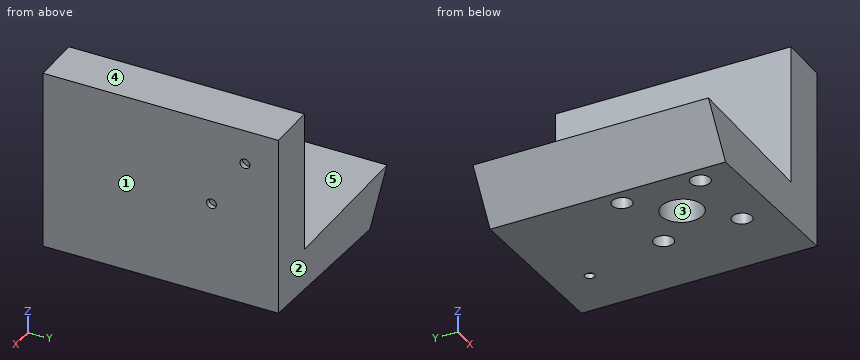
from build123d import *

# Parameters (mm, degrees)
SKETCH1_W           = 41.85
SKETCH1_H           = 10
SKETCH1_W_2         = 10
SKETCH1_H_2         = 29
BOSS_EXTRUDE1_DEPTH = 48
CUT_EXTRUDE1_DEPTH  = 48
SKETCH4_R           = 2
SKETCH4_R_2         = 4.2
CUT_EXTRUDE2_DEPTH  = 48
CUT_EXTRUDE3_DEPTH  = 48
SKETCH6_R           = 1
CUT_EXTRUDE4_DEPTH  = 2
SKETCH7_R           = 1
CUT_EXTRUDE5_DEPTH  = 1
SKETCH8_W           = 65.86504954
SKETCH8_H           = 108.734415267
CUT_EXTRUDE6_DEPTH  = 17.96
BOSS_EXTRUDE2_DEPTH = 17.96
SKETCH10_R          = 1
CUT_EXTRUDE7_DEPTH  = 1
SKETCH11_R          = 1
CUT_EXTRUDE8_DEPTH  = 1


with BuildPart() as part:
    # Sketch1 → Boss-Extrude1 (new body)
    with BuildSketch(Plane(origin=(0, 0, 0), x_dir=(1, 0, 0), z_dir=(0, 1, 0))):
        with Locations((-10.925, 5)):
            Rectangle(SKETCH1_W, SKETCH1_H)
        with Locations((5, -14.5)):
            Rectangle(SKETCH1_W_2, SKETCH1_H_2)
    extrude(amount=BOSS_EXTRUDE1_DEPTH)

    # Sketch3 → Cut-Extrude1 (cut)
    with BuildSketch(Plane(origin=(0, 48, 0), x_dir=(1, 0, 0), z_dir=(0, 1, 0))):
        Polygon((-31.85, 10), (-25.26317425, 10), (-31.85, 0), align=None)
    extrude(amount=-CUT_EXTRUDE1_DEPTH, mode=Mode.SUBTRACT)

    # Sketch4 → Cut-Extrude2 (cut)
    with BuildSketch(Plane.XY):
        with Locations((-5.589559388, 40.980827232)):
            Circle(SKETCH4_R)
        with Locations((-5.629681083, 24.979051073)):
            Circle(SKETCH4_R)
        with Locations((-21.591335547, 41.020948927)):
            Circle(SKETCH4_R)
        with Locations((-21.631457243, 25.019172768)):
            Circle(SKETCH4_R)
        with Locations((-13.629681083, 32.979051073)):
            Circle(SKETCH4_R_2)
    extrude(amount=-CUT_EXTRUDE2_DEPTH, mode=Mode.SUBTRACT)

    # Sketch5 → Cut-Extrude3 (cut)
    with BuildSketch(Plane(origin=(0, 48, 0), x_dir=(1, 0, 0), z_dir=(0, 1, 0))):
        Polygon((-25.26317425, 10), (10, 8), (10, 10), align=None)
    extrude(amount=-CUT_EXTRUDE3_DEPTH, mode=Mode.SUBTRACT)

    # Sketch6 → Cut-Extrude4 (cut)
    with BuildSketch(Plane(origin=(10, 0, 0), x_dir=(0, 0, -1), z_dir=(1, 0, 0))):
        with Locations((-21, 6.391948522)):
            Circle(SKETCH6_R)
        with Locations((-11, 15)):
            Circle(SKETCH6_R)
    extrude(amount=-CUT_EXTRUDE4_DEPTH, mode=Mode.SUBTRACT)

    # Sketch7 → Cut-Extrude5 (cut)
    with BuildSketch(Plane(origin=(0.484340621, 0, -8.539693864), x_dir=(-0.9983954953921488, 0, -0.056625389894163713), z_dir=(0.056625389894163713, 0, -0.9983954953921488))):
        with Locations((10.469048165, 7)):
            Circle(SKETCH7_R)
    extrude(amount=-CUT_EXTRUDE5_DEPTH, mode=Mode.SUBTRACT)

    # Sketch8 → Cut-Extrude6 (cut)
    with BuildSketch(Plane.XZ):
        with Locations((-12.632558392, 5.858470362)):
            Rectangle(SKETCH8_W, SKETCH8_H)
    extrude(amount=-CUT_EXTRUDE6_DEPTH, mode=Mode.SUBTRACT)

    # Sketch9 → Boss-Extrude2 (add)
    with BuildSketch(Plane(origin=(0, 48, 0), x_dir=(1, 0, 0), z_dir=(0, 1, 0))):
        Polygon((10, -29), (0, -29), (0, 0), (-31.85, 0), (-25.26317425, 10), (10, 8), align=None)
    extrude(amount=BOSS_EXTRUDE2_DEPTH)

    # Sketch10 → Cut-Extrude7 (cut)
    with BuildSketch(Plane(origin=(10, 0, 0), x_dir=(0, 0, -1), z_dir=(1, 0, 0))):
        with Locations((-21.942879274, 59.132798009)):
            Circle(SKETCH10_R)
        with Locations((-11.347569505, 52.312182855)):
            Circle(SKETCH10_R)
    extrude(amount=-CUT_EXTRUDE7_DEPTH, mode=Mode.SUBTRACT)

    # Sketch11 → Cut-Extrude8 (cut)
    with BuildSketch(Plane(origin=(0.484340621, 0, -8.539693864), x_dir=(-0.9983954953921488, 0, -0.056625389894163713), z_dir=(0.056625389894163713, 0, -0.9983954953921488))):
        with Locations((1.733457751, 58.349902704)):
            Circle(SKETCH11_R)
    extrude(amount=-CUT_EXTRUDE8_DEPTH, mode=Mode.SUBTRACT)


solid = part.part
Geometry: final body of the model. Coordinates: model frame, mm. Face numbers are marked on the shaded views. A direction names the side the tool comes from. Coordinates: 2 decimals unless noted, no trailing zeros. Order: outer loops, then holes, each group sorted by start corner. A loop starts at its lowest first (then second) coordinate and runs counter-clockwise, first axis right, second up.
(1) Draft query along X for the marked faces 1, 2 and 3. Return one class per face: pulls with the +X half, pulls with the -X half, needs draft (parallel to the pull), parting line crosses it, or undercut.
(2) Material intervals for probe 1 along X at (y, z) = (25, -6); probe 2 along X at (y, z) = (24.5, 18); probe 3 along Y at (x, z) = (-15.5, -1.5), sorted ascending.
(3) Section query C-C (y = 50.5). Return the cut outline in (x, z).
(4) Section query D-D (z = 2). Return the cut outline in (x, y).
(5) Access query for the marked faces 4 and 5. Directions: +Z, -Z, +X, -X, +Y, -Y. A direction counts if a zero-diameter tool reaches every point of the face in a straight line with its end or side. Return the directions, or none.
(6) Section query A-A (x = -11). Return the cut outline in (y, z).
(7) Section query B-B (y = 29.5). Return the cut outline in (x, z).
(8) First-contact query: pin 1 (5 mm diameter, centred on x = -21.63, y = 25.02, fed in from -Z); pin 2 (10 mm diameter, centred on y = 45.5, z = 23.5, fed in from -X); pin 3 (4.5 mm diameter, centred on x = -5.59, y = 40.98, fed in from -Z). Flat tips, straight axial feed; report the tip coordinate or a pass-through.
Solution:
1. face 1: pulls with the +X half
1. face 2: needs draft
1. face 3: undercut
2. probe 1: x = -27.9 to -23.63, -19.63 to -7.63, -3.63 to 10
2. probe 2: x = 0 to 10
2. probe 3: y = 17.96 to 29.22, 36.74 to 65.96
3. outline: (-31.85, 0) - (-25.26, -10) - (10, -8) - (10, 29) - (0, 29) - (0, 0) - close
4. outline: (0, 17.96) - (10, 17.96) - (10, 65.96) - (0, 65.96) - close
5. face 4: +Z, +X, -X, +Y, -Y
5. face 5: +Z, -X, +Y, -Y
6. outline: (17.96, -9.19) - (29.7, -9.19) - (29.7, 0) - (17.96, 0) - close; (36.25, -9.19) - (65.96, -9.19) - (65.96, 0) - (36.25, 0) - close
7. outline: (-31.85, 0) - (-25.26, -10) - (-15.98, -9.47) - (-15.98, 0) - close; (-11.28, -9.21) - (10, -8) - (10, 29) - (0, 29) - (0, 0) - (-11.28, 0) - close
8. pin 1: stops at z = -9.94
8. pin 2: stops at x = 0
8. pin 3: stops at z = -9.01
